Autodesk Inventor part; units mm, degrees
ref_plane "YZ Plane" through (0, 0, 0) normal (1, 0, 0) x (0, 1, 0)
ref_plane "XZ Plane" through (0, 0, 0) normal (0, 1, 0) x (-1, 0, 0)
ref_plane "XY Plane" through (0, 0, 0) normal (0, 0, 1) x (1, 0, 0)
sketch "Sketch_1" plane through (0, 0, 0) normal (0, 0, 1) x (1, 0, 0)
  line L0 (8, 0) -> (-7.8, 0)
  line L1 (-7.8, 0) -> (-7.8, 5)
  line L2 (-7.8, 5) -> (-5, 5)
  line L3 (-5, 5) -> (-5, 3)
  line L4 (-5, 3) -> (0, 3)
  line L5 (0, 3) -> (0, 2)
  line L6 (0, 2) -> (7.5705, 2)
  line L7 (7.5705, 2) -> (8, 1.5705)
  line L8 (8, 1.5705) -> (8, 0)
  line L9 (8, 0) -> (-7.8, 0)
revolve "Revolution1" add sketch "Sketch_1" angle 360 about axis through (8, 0, 0) along (1, 0, 0)
thread "Thread1"
sketch "Sketch_2" plane through (-7.8, 0, 0) normal (-1, 0, 0) x (0, 1, 0)
  line L0 (-1.4434, 0) -> (-0.7217, -1.25)
  line L1 (-0.7217, -1.25) -> (0.7217, -1.25)
  line L2 (0.7217, -1.25) -> (1.4434, 0)
  line L3 (1.4434, 0) -> (0.7217, 1.25)
  line L4 (0.7217, 1.25) -> (-0.7217, 1.25)
  line L5 (-0.7217, 1.25) -> (-1.4434, 0)
extrude "Extrusion1" cut sketch "Sketch_2" against normal blind 2.5
sketch "Sketch_3" plane through (0, 0, 0) normal (0, 0, 1) x (1, 0, 0)
  line L0 (-4.5783, 0) -> (-5.3, 0)
  line L1 (-5.3, 0) -> (-5.3, 1.25)
  line L2 (-5.3, 1.25) -> (-4.5783, 0)
  line L3 (-4.5783, 0) -> (-5.3, 0)
revolve "Revolution2" cut sketch "Sketch_3" angle 360 about axis through (-4.5783, 0, 0) along (1, 0, 0)
properties part number "DBSY4-5-8" material "스테인리스스틸"
Design review of the part built by this model. Coordinates are the model's own, in mm. A direction names the side the tool comes from. Give positions to 0.01 mm unless a question says otherwise; leave off trailing zeros. Order: outer loops, then holes, each group sorted by start corner. A loop starts at its lowest first (then second) coordinate and runs counter-clockwise, first axis right, second up. Notation, with made-up numbers: (48.5, 89) -> (101.5, 89) arc R18 ccw to (101.5, 102) -> close; hole circle Ø9 at (37, 58). An arc over 180 degrees is marked (long way). Write each question's results on one line, items separated by ' | '. Start each with the question number.
Q1. Wall thickness on L1, parallel to X at y = -1.25, z = 4.25; L2, parallel to X at y = 2, z = 1.5; L3, parallel to Z at x = 7.25, y = 1.25: over which ranges is each line inside the solid? List them lowest first. Write a range as from..to.
Q2. Add section A-A on y = -4. Give the boundary of the cut face in (x, z), and give its area (3 significant figures).
Q3. For pin 1 (5 mm diameter, centred on x = 5, y = 3, fed in from +Z); pin 2 (2 mm diameter, centred on x = 4, z = 0, fed in from -Y); pin 3 (3 mm diameter, centred on x = 0, y = 0, fed in from +Z), all flat-tipped, find the tip position at first contact; note any pin that passes through.
Q4. Mouldability with a two-part tool opening along Y and no side actions: class faces 1 (the flat face through (-6.57, 1.08, 0.63)), 2 (the flat face through (8, 0, 0)), 3 (the cylindrical face through (-6.38, -1.08, -4.88)) as +Y half, -Y half, draft (parallel to the pull), parting line (faces both ways), or undercut.
Q5. Machinability: for faces 4 (the flat face through (-7, 0, -1.25)), 5 (the flat face through (-7.8, 1.04, -1.04)), 6 (the flat face through (0, 1, -2)), which of the approach directions +Z, -Z, +X, -X, +Y, -Y give a long, thin tool a straight path to every point of the face, cutting with its end or side? Answer none if there is none.
Q6. Add section B-B on x = 5. Give the boundary of the cut face in (y, z).
Found:
1) L1: x = -7.8..-5 | L2: x = -7.8..0 | L3: z = -1.56..1.56
2) outline: (-7.8, -3) -> (-5, -3) -> (-5, 3) -> (-7.8, 3) -> close | area: 16.8 mm2
3) pin 1: stops at z = 1.94 | pin 2: stops at y = -2 | pin 3: stops at z = 3
4) face 1: undercut | face 2: draft | face 3: parting line
5) face 4: -X | face 5: +Z, -Z, -X, +Y, -Y | face 6: +X
6) outline: circle Ø4 at (0, 0)
